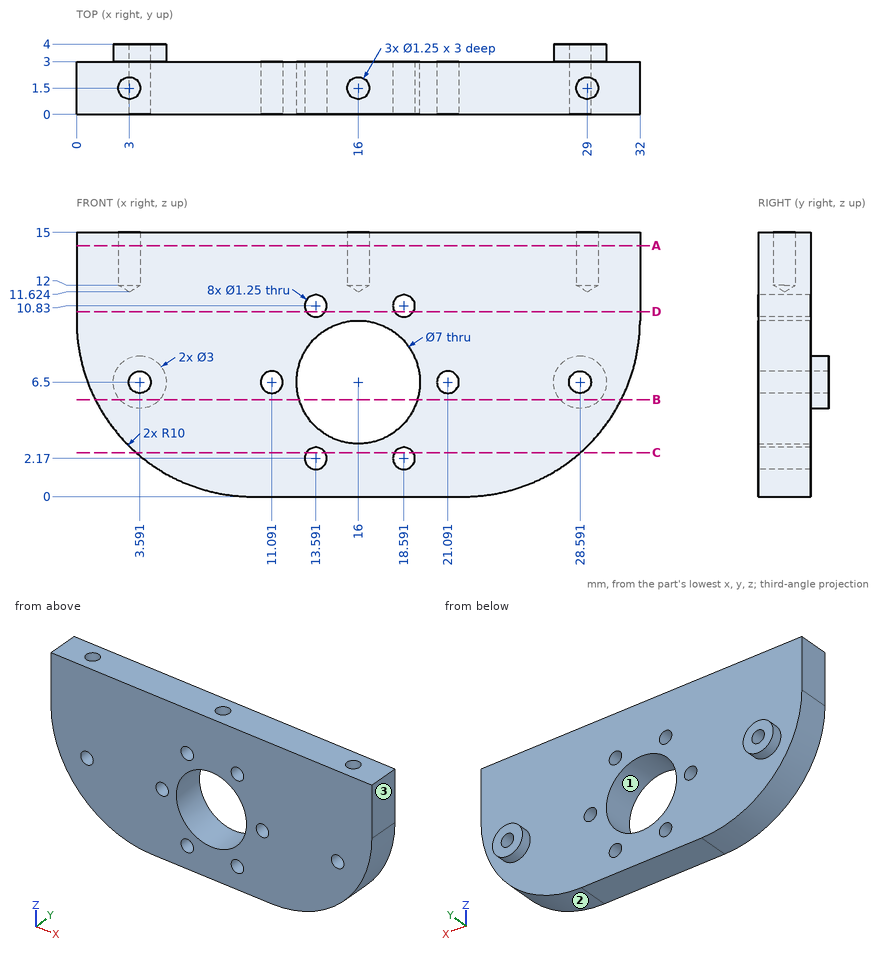
Input: dimensioned drawing with shaded views. Units: mm. Origin: part minimum x, y, z. Coordinates: 2 decimals unless noted, no trailing zeros. Write each loop counter-clockwise with the first axis right and the second up, starting at its lowest first coordinate (ties: lowest second). Pieces come first, ordered by that corner, then holes. Notation, with made-up numbers: (-11, -3) -> (24, -3) arc R13 ccw to (24, 6) -> close; hole circle Ø2 at (-8.75, -34.75). An arc over 180 degrees is marked (long way). Return JSON: item names as keys, results as strings. Group by question number.
1) Section query C-C, the plane z = 2.5. Return loops of the section in (x, y) (1 decimal).
2) Contact query for flat-ended pins moving along their axis: P1, Ø4.5, axis at x = 16, z = 9, coming from the +Y side; P2, Ø8, axis at x = 16, z = 6.5, coming from the -Y side; P3, Ø2, axis at x = 29, y = 1.5, coming from the -Z side; P4, Ø0.8, axis at x = 18.59, z = 10.83, coming from the -Y side. Output: stop coordinate, or through.
3) Section query B-B, the plane z = 5.5. Return loops of the section in (x, y) (1 decimal).
4) Section query D-D, the plane z = 10.5. Return loops of the section in (x, y).
5) Ray query, line 1 along X through (y, z) = (2.7, 6) (1 decimal); line 2 along Y through (x, z) = (16, 13.7) (1 decimal); line 3 along Z through (x, y) = (14, 0.4) (1 decimal). Return the intervals inside material, ascending.
6) Mould query, pull axis Z, two halves, no side actions, for the marked faces 1, 2 and 3. Classes: +Z half, -Z half, draft (parallel to the pull), parting line (faces both ways), or undercut.
7) Section query A-A, the plane z = 14.25. State how many separate pieces and enclosed holes the cut face has.
From the geometry:
{
 "1": {"outline": "(3.4, 0) -> (13.1, 0) -> (13.1, 3) -> (3.4, 3) -> close; (14.1, 0) -> (18.1, 0) -> (18.1, 3) -> (14.1, 3) -> close; (19.1, 0) -> (28.6, 0) -> (28.6, 3) -> (19.1, 3) -> close"},
 "2": {"P1": "y = 3", "P2": "y = 0", "P3": "z = 2", "P4": "through"},
 "3": {"outline": "(1.1, 0) -> (12.6, 0) -> (12.6, 3) -> (4.7, 3) -> (4.7, 4) -> (2.5, 4) -> (2.5, 3) -> (1.1, 3) -> close; (19.4, 0) -> (30.9, 0) -> (30.9, 3) -> (29.7, 3) -> (29.7, 4) -> (27.5, 4) -> (27.5, 3) -> (19.4, 3) -> close"},
 "4": {"outline": "(0, 0) -> (13.06, 0) -> (13.06, 3) -> (0, 3) -> close; (14.12, 0) -> (18.06, 0) -> (18.06, 3) -> (14.12, 3) -> close; (19.12, 0) -> (32, 0) -> (32, 3) -> (19.12, 3) -> close"},
 "5": {"line 1": "0.8 to 3.2, 4 to 10.7, 11.5 to 12.5, 19.5 to 20.7, 21.5 to 28.2, 29 to 31.2", "line 2": "0 to 0.9, 2.1 to 3", "line 3": "0 to 1.7, 2.6 to 3.6, 9.4 to 10.4, 11.3 to 15"},
 "6": {"face 1": "undercut", "face 2": "-Z half", "face 3": "draft"},
 "7": {"separate pieces": "1", "enclosed holes": "3"}
}
